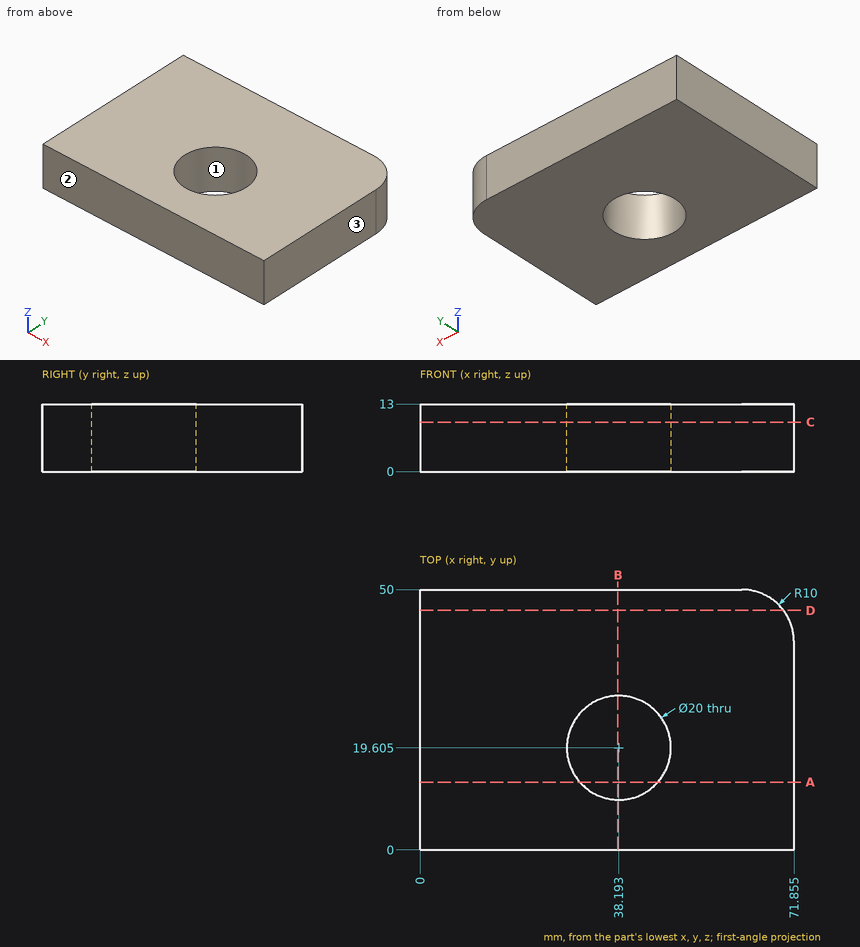
Here's the drawing with two shaded views (mm, measured from the low corner). I have some questions. Round coordinates to 2 decimals unless told otherwise and drop trailing zeros. Loops run counter-clockwise (first coordinate to the right, second up) from the corner with the lowest first, then second, coordinate; pieces in that order, holes last. Notation, with made-up numbers: (88, 16.25) - (103, 16.25) arc R10 cw to (103, 25.25) - close; hole circle Ø8 at (17, 51). An arc over 180 degrees is marked (long way). Use CSV: the item, a comma, the result in double quotes.
Item 1: If we section it at C-C on z = 9.5: List the corners of the cut face in (x, y) for me (1 decimal), then the cut area to 3 significant figures.
Here are the results:
outline,"(0, 0) - (71.9, 0) - (71.9, 40) arc R10 ccw to (61.9, 50) - (0, 50) - close; hole circle Ø20 at (38.2, 19.6)"
area,"3,260 mm²"
Item 2: I need wall thicknesses on L1, parallel to Y at x = 38, z = 5; L2, parallel to X at y = 15, z = 12.75 (1 decimal); L3, parallel to X at y = 42.5, z = 8. Which ranges of each line are inside material? Lowest first, please. Write a range as [from, to].
Here are the results:
L1,"y = [0, 9.61], [29.6, 50]"
L2,"x = [0, 29.3], [47.1, 71.9]"
L3,"x = [0, 71.54]"
Item 3: If we section it at D-D on y = 46: List the corners of the cut face in (x, z) for me (1 decimal), then the cut area to 3 significant figures.
Here are the results:
outline,"(0, 0) - (69.9, 0) - (69.9, 13) - (0, 13) - close"
area,"908 mm²"
Item 4: Will this pin go through, and if not, where does the flat tip stop? pin 1 (18 mm diameter, centred on x = 38.19, y = 19.6, fed in from -Z).
Here are the results:
pin 1,"passes through"
Item 5: If we section it at A-A on y = 13: List the corners of the cut face in (x, z) for me (1 decimal).
Here are the results:
outline,"(0, 0) - (30.7, 0) - (30.7, 13) - (0, 13) - close; (45.7, 0) - (71.9, 0) - (71.9, 13) - (45.7, 13) - close"
Item 6: If we mould it in two halves opening along Y, with no side actions, what happens to the marked faces 1, 2 and 3? For each: pulls with the +Y half, pulls with the -Y half, needs draft (parallel to the pull), parting line crosses it, or undercut.
Here are the results:
face 1,"undercut"
face 2,"pulls with the -Y half"
face 3,"needs draft"
Item 7: If we section it at B-B on x = 38: List the corners of the cut face in (y, z) for me, then the cut area to 3 significant figures.
Here are the results:
outline,"(0, 0) - (9.61, 0) - (9.61, 13) - (0, 13) - close; (29.6, 0) - (50, 0) - (50, 13) - (29.6, 13) - close"
area,"390 mm²"
